from build123d import *

# Parameters (mm, degrees)
SKETCH1_W                = 74.549
SKETCH1_H                = 74.549
SKETCH1_R                = 24.511
BOSS_EXTRUDE1_DEPTH      = 1.5748
BOSS_EXTRUDE1_DEPTH_BACK = 1.5875
SKETCH2_R                = 3.429
CUT_EXTRUDE1_DEPTH       = 4.1623
BOSS_EXTRUDE2_DEPTH      = 0.0508
FILLET3_R                = 2.54
FILLET3_OF_MIRROR3_R     = 2.54
MIRROR2_COPY_1_SKETCH_R  = 3.429
MIRROR2_COPY_1_DEPTH     = 4.1623
SKETCH14_W               = 42.799
SKETCH14_H               = 8.290530285
CUT_EXTRUDE2_DEPTH       = 4.1623
FILLET1_R                = 2.54
SKETCH17_W               = 14.315330836
SKETCH17_H               = 49.149
CUT_EXTRUDE3_DEPTH       = 4.1623
FILLET2_R                = 2.54
FILLET5_R                = 2.54


with BuildPart() as part:
    # Sketch1 → Boss-Extrude1 (new body, two sides)
    with BuildSketch(Plane.XY) as boss_extrude1_sk:
        Rectangle(SKETCH1_W, SKETCH1_H)
        Circle(SKETCH1_R, mode=Mode.SUBTRACT)
    extrude(amount=BOSS_EXTRUDE1_DEPTH)
    extrude(boss_extrude1_sk.sketch, amount=-BOSS_EXTRUDE1_DEPTH_BACK)

    # Sketch2 → Cut-Extrude1 (cut, through all)
    with BuildSketch(Plane.XY.offset(1.5748)):
        with Locations((-31.75, 31.75)):
            Circle(SKETCH2_R)
    cut_extrude1 = extrude(amount=-CUT_EXTRUDE1_DEPTH, mode=Mode.SUBTRACT)

    # Sketch20 → Boss-Extrude2 (add)
    with BuildSketch(Plane.XY.offset(1.5748)):
        Polygon((-24.921174252, 24.5745), (-24.921174252, 30.9245), (-18.2245, 30.9245), (-18.2245, 37.2745), (-27.1145, 37.2745), (-27.1145, 27.1145), (-34.7345, 27.1145), (-34.7345, 0), (-32.1945, 0), (-32.1945, 24.5745), align=None)
    boss_extrude2 = extrude(amount=BOSS_EXTRUDE2_DEPTH)

    # Fillet3
    fillet3_edges = [part.edges().sort_by_distance(p)[0] for p in [
        (-34.7345, 27.1145, 1.6002),
        (-32.1945, 24.5745, 1.6002),
        (-18.2245, 30.9245, 1.6002),
        (-24.921174252, 24.5745, 1.6002),
        (-24.921174252, 30.9245, 1.6002),
    ]]
    fillet(fillet3_edges, radius=FILLET3_R)

    # Mirror3: Boss-Extrude2 across plane
    add(boss_extrude2.mirror(Plane.ZX))

    # Fillet3 of Mirror3
    fillet3_of_mirror3_edges = [part.edges().sort_by_distance(p)[0] for p in [
        (-34.7345, -27.1145, 1.6002),
        (-32.1945, -24.5745, 1.6002),
        (-18.2245, -30.9245, 1.6002),
        (-24.921174252, -24.5745, 1.6002),
        (-24.921174252, -30.9245, 1.6002),
    ]]
    fillet(fillet3_of_mirror3_edges, radius=FILLET3_OF_MIRROR3_R)

    # Mirror1: Cut-Extrude1 across plane
    add(cut_extrude1.mirror(Plane(origin=(0, 0, 0), x_dir=(0, 0, 1), z_dir=(1, 0, 0))), mode=Mode.SUBTRACT)

    # Mirror2: Cut-Extrude1 across plane
    add(cut_extrude1.mirror(Plane.ZX), mode=Mode.SUBTRACT)

    # Mirror2 copy 1 sketch → Mirror2 copy 1 (cut, through all)
    with BuildSketch(Plane(origin=(0, 0, 1.5748), x_dir=(-1, 0, 0), z_dir=(0, 0, 1))):
        with Locations((-31.75, 31.75)):
            Circle(MIRROR2_COPY_1_SKETCH_R)
    extrude(amount=-MIRROR2_COPY_1_DEPTH, mode=Mode.SUBTRACT)

    # Sketch14 → Cut-Extrude2 (cut, through all)
    with BuildSketch(Plane.XY.offset(1.5748)):
        with Locations((3.175, 35.069765143)):
            Rectangle(SKETCH14_W, SKETCH14_H)
    extrude(amount=-CUT_EXTRUDE2_DEPTH, mode=Mode.SUBTRACT)

    # Fillet1
    fillet1_edges = [part.edges().sort_by_distance(p)[0] for p in [
        (-18.2245, 30.9245, -0.00635),
        (24.5745, 30.9245, -0.00635),
    ]]
    fillet(fillet1_edges, radius=FILLET1_R)

    # Sketch17 → Cut-Extrude3 (cut, through all)
    with BuildSketch(Plane.XY.offset(1.5748)):
        with Locations((34.907165418, 0)):
            Rectangle(SKETCH17_W, SKETCH17_H)
    extrude(amount=-CUT_EXTRUDE3_DEPTH, mode=Mode.SUBTRACT)

    # Fillet2
    fillet2_edges = [part.edges().sort_by_distance(p)[0] for p in [
        (27.7495, -24.5745, -0.00635),
        (27.7495, 24.5745, -0.00635),
    ]]
    fillet(fillet2_edges, radius=FILLET2_R)

    # Fillet5
    fillet5_edges = [part.edges().sort_by_distance(p)[0] for p in [
        (-27.1145, -27.1145, 1.6002),
        (-27.1145, 27.1145, 1.6002),
    ]]
    fillet(fillet5_edges, radius=FILLET5_R)


solid = part.part
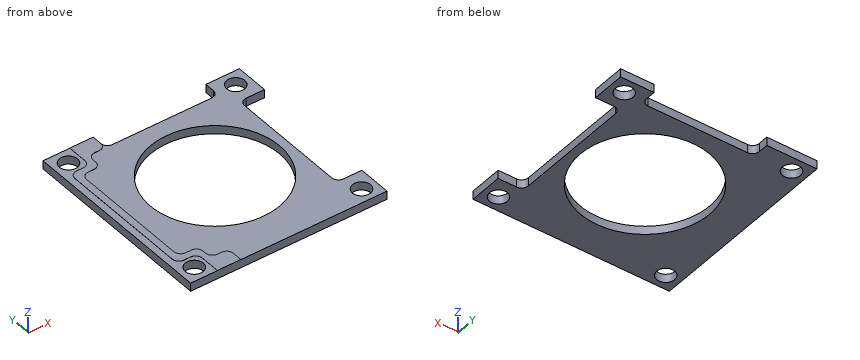
CAD build for the part. Positions are in the model's coordinates, mm. Give positions to 0.01 mm unless a question says otherwise; leave off trailing zeros. Loops run counter-clockwise (first coordinate to the right, second up) from the corner with the lowest first, then second, coordinate; pieces in that order, holes last. Notation, with made-up numbers: M 43,-4 L 84,-4 A29 cw 84,31 Z; hole C -2,83 d8. An arc over 180 degrees is marked long. Answer in a Markdown table with one row per item. Add a question column.
Item 1: Drop flat-ended pins along their axis: P1, Ø8, axis at x = -26, y = -1, coming from the +Z side; P2, Ø1.5, axis at x = -10, z = 1, coming from the +Y side. Give the stop position or say it passes through.
Item 2: Band-saw the part on B-B on y = 0. Give the cut face in (x, z), then the cut area to 3 significant figures.
Item 3: Probe probe 1 along Y at (x, z) = (-31.75, -0.2); probe 2 along X at (y, z) = (-33.5, 1.4); probe 3 along Z at (x, y) = (18, -24). List the from-to ranges inside material, lowest first.
Item 4: Band-saw the part on D-D on x = -11.5. Give the cut face in (y, z).
Item 5: Band-saw the part on C-C on z = -0.2. Give the cut face in (x, y), then the cut area to 3 significant figures.
Item 6: Band-saw the part on A-A on x = 31.75. Give the cut face in (y, z), then the cut area to 3 significant figures.
Reply:
| question | item | result |
|---|---|---|
| 1 | P1 | stops at z = 1.57 |
| 1 | P2 | stops at y = 30.92 |
| 2 | outline | M -37.27,-1.59 L -24.51,-1.59 L -24.51,1.57 L -32.19,1.57 L -32.19,1.63 L -34.73,1.63 L -34.73,1.57 L -37.27,1.57 Z; M 24.51,-1.59 L 27.75,-1.59 L 27.75,1.57 L 24.51,1.57 Z |
| 2 | area | 50.7 mm^2 |
| 3 | probe 1 | y = -37.27 to -35.18, -28.32 to 28.32, 35.18 to 37.27 |
| 3 | probe 2 | x = -37.27 to -34.7, -28.8 to 28.8, 34.7 to 37.27 |
| 3 | probe 3 | z = -1.59 to 1.57 |
| 4 | outline | M -37.27,-1.59 L -21.65,-1.59 L -21.65,1.57 L -37.27,1.57 Z; M 21.65,-1.59 L 30.92,-1.59 L 30.92,1.57 L 21.65,1.57 Z |
| 5 | outline | M -37.27,-37.27 L 37.27,-37.27 L 37.27,-24.57 L 30.29,-24.57 A2.54 cw 27.75,-22.03 L 27.75,22.03 A2.54 cw 30.29,24.57 L 37.27,24.57 L 37.27,37.27 L 24.57,37.27 L 24.57,33.46 A2.54 cw 22.03,30.92 L -15.68,30.92 A2.54 cw -18.22,33.46 L -18.22,37.27 L -37.27,37.27 Z; hole C -31.75,-31.75 d6.86; hole C -31.75,31.75 d6.86; hole C 0,0 d49.02; hole C 31.75,-31.75 d6.86; hole C 31.75,31.75 d6.86 |
| 5 | area | 2,790 mm^2 |
| 6 | outline | M -37.27,-1.59 L -35.18,-1.59 L -35.18,1.57 L -37.27,1.57 Z; M -28.32,-1.59 L -24.57,-1.59 L -24.57,1.57 L -28.32,1.57 Z; M 24.57,-1.59 L 28.32,-1.59 L 28.32,1.57 L 24.57,1.57 Z; M 35.18,-1.59 L 37.27,-1.59 L 37.27,1.57 L 35.18,1.57 Z |
| 6 | area | 36.9 mm^2 |
